from build123d import *

# Parameters (mm, degrees)
BOSS_EXTRUDE1_DEPTH = 50
SKETCH2_W           = 30
SKETCH2_H           = 30
CUT_EXTRUDE1_DEPTH  = 65
SKETCH3_R           = 7.5
CUT_EXTRUDE2_DEPTH  = 40
SKETCH4_R           = 20
BOSS_EXTRUDE2_DEPTH = 30
CUT_EXTRUDE3_START  = -15
CUT_EXTRUDE3_DEPTH  = 15


with BuildPart() as part:
    # Sketch1 → Boss-Extrude1 (new body)
    with BuildSketch(Plane.XY):
        Polygon((0, 0), (-15, 0), (-15, 10), (-45, 10), (-45, 20), (-27.5, 70), (27.5, 70), (45, 20), (45, 10), (15, 10), (15, 0), align=None)
    extrude(amount=BOSS_EXTRUDE1_DEPTH)

    # Sketch2 → Cut-Extrude1 (cut, symmetric)
    with BuildSketch(Plane(origin=(0, 0, 0), x_dir=(0, 0, -1), z_dir=(1, 0, 0))):
        with Locations((-25, 46)):
            Rectangle(SKETCH2_W, SKETCH2_H)
    extrude(amount=CUT_EXTRUDE1_DEPTH, both=True, mode=Mode.SUBTRACT)

    # Sketch3 → Cut-Extrude2 (cut)
    with BuildSketch(Plane(origin=(0, 0, 0), x_dir=(1, 0, 0), z_dir=(0, 1, 0))):
        with Locations(Location((-31.15, -25, 0), (0, 0, 90))):
            Circle(SKETCH3_R)
        with Locations(Location((31.15, -25, 0), (0, 0, 90))):
            Circle(SKETCH3_R)
    extrude(amount=CUT_EXTRUDE2_DEPTH, mode=Mode.SUBTRACT)

    # Sketch4 → Boss-Extrude2 (add)
    with BuildSketch(Plane(origin=(0, 70, 0), x_dir=(1, 0, 0), z_dir=(0, 1, 0))):
        with Locations(Location((0, -25, 0), (0, 0, 90))):
            Circle(SKETCH4_R)
    extrude(amount=BOSS_EXTRUDE2_DEPTH)

    # Sketch5 → Cut-Extrude3 (cut)
    with BuildSketch(Plane(origin=(0, 100, 0), x_dir=(1, 0, 0), z_dir=(0, 1, 0)).offset(CUT_EXTRUDE3_START)):
        with BuildLine():
            ThreePointArc((18.33030278, -17), (0, -5), (-18.33030278, -17))
            Line((-18.33030278, -17), (18.33030278, -17))
        make_face()
        with BuildLine():
            Line((18.33030278, -33), (-18.33030278, -33))
            ThreePointArc((-18.33030278, -33), (0, -45), (18.33030278, -33))
        make_face()
    extrude(amount=CUT_EXTRUDE3_DEPTH, mode=Mode.SUBTRACT)


solid = part.part
Could you check a few things on this model? Use its own coordinates, in mm. A direction names the side the tool comes from. Give positions to 0.01 mm unless a question says otherwise; leave off trailing zeros. Write each loop counter-clockwise with the first axis right and the second up, starting at its lowest first coordinate (ties: lowest second). Pieces come first, ordered by that corner, then holes. Notation, with made-up numbers: (-11.75, -32.75) - (1.25, -32.75) arc R16 cw to (1.25, -2.75) - close; hole circle Ø9 at (34, 85.5). An arc over 180 degrees is marked (long way). Use CSV: the item, a comma, the result in double quotes. Start each with the question number.
Item 1: I want a section at C-C, the plane z = 25. Please give me the cut outline in (x, y), then the cut area to 3 significant figures.
Item 2: I'm going to push flat-ended pins straight in: pin 1 (8 mm diameter, centred on x = 6.5, z = 39, fed in from +Y); pin 2 (3 mm diameter, centred on y = 6.5, z = 19, fed in from +X); pin 3 (16.5 mm diameter, centred on x = 7.5, y = 89, fed in from -Z). Where does each tip first touch, or does it pass through?
Item 3: I want a section at D-D, the plane y = 14.5. Please give me the cut outline in (x, z), then the cut area to 3 significant figures.
Item 4: If I drill on line 1 along Y through (x, z) = (20, 28.5); line 2 along Y through (x, z) = (-8, 33.5); line 3 along X through (y, z) = (26.25, 25), over which ranges is the centre line in solid material (lowest first)?
Item 5: If we mould it in two halves opening along Z, with no side actions, what happens to faces 1 (the face through (26.081, 20.353, 30.528)), 2 (the face through (-0.88, 81.46, 44.98)), 3 (the face through (36.128, 45.35, 41.317))? For each: pulls with the +Z half, pulls with the -Z half, needs draft (parallel to the pull), parting line crosses it, or undercut.
Item 6: I want a section at A-A, the plane x = 0. Please give me the cut outline in (y, z), then the cut area to 3 significant figures.
Item 7: I want a section at B-B, the plane y = 59. Please give me the cut outline in (x, z).
Item 8: For faces 4 (the face through (1, 31, 25)), 5 (the face through (0, 85, 12)), 6 (the face through (-26, 10, 19)), 7 (the face through (15, 5, 25)), which set-ups out of +Z, -Z, +X, -X, +Y, -Y let a thin tool reach every point of the face, with its end or its side?
Findings:
1,outline,"(-45, 10) - (-38.65, 10) - (-38.65, 31) - (-41.15, 31) - (-45, 20) - close; (-30.65, 61) - (30.65, 61) - (27.5, 70) - (20, 70) - (20, 100) - (-20, 100) - (-20, 70) - (-27.5, 70) - close; (-23.65, 10) - (-15, 10) - (-15, 0) - (15, 0) - (15, 10) - (23.65, 10) - (23.65, 31) - (-23.65, 31) - close; (38.65, 10) - (45, 10) - (45, 20) - (41.15, 31) - (38.65, 31) - close"
1,area,"3,240 mm2"
2,pin 1,"stops at y = 85"
2,pin 2,"stops at x = 15"
2,pin 3,"stops at z = 5"
3,outline,"(-45, 0) - (45, 0) - (45, 50) - (-45, 50) - close; hole circle Ø15 at (-31.15, 25); hole circle Ø15 at (31.15, 25)"
3,area,"4,150 mm2"
4,line 1,"y = 10 to 31, 61 to 70"
4,line 2,"y = 0 to 31, 61 to 85"
4,line 3,"x = -42.81 to -38.65, -23.65 to 23.65, 38.65 to 42.81"
5,face 1,"undercut"
5,face 2,"parting line crosses it"
5,face 3,"needs draft"
6,outline,"(0, 0) - (70, 0) - (70, 5) - (85, 5) - (85, 17) - (100, 17) - (100, 33) - (85, 33) - (85, 45) - (70, 45) - (70, 50) - (0, 50) - close; hole (31, 10) - (61, 10) - (61, 40) - (31, 40) - close"
6,area,"3,440 mm2"
7,outline,"(-31.35, 0) - (31.35, 0) - (31.35, 10) - (-31.35, 10) - close; (-31.35, 40) - (31.35, 40) - (31.35, 50) - (-31.35, 50) - close"
8,face 4,"+X, -X"
8,face 5,"-Z, +X, -X, +Y"
8,face 6,"+Z, -Z, -X, -Y"
8,face 7,"+Z, -Z, +X, -Y"
